```python
from build123d import *

# Parameters (mm, degrees)
BOSS_EXTRUDE1_DEPTH = 15.5
FILLET1_R           = 0.2
FILLET2_R           = 0.2
FILLET3_R           = 0.2


with BuildPart() as part:
    # Sketch1 → Boss-Extrude1 (new body)
    with BuildSketch(Plane(origin=(0, 0, 0), x_dir=(1, 0, 0), z_dir=(0, 1, 0))):
        Polygon((-0.9, 0.9), (-0.9, 2.35), (0.9, 2.35), (0.9, 0.9), (2.35, 0.9), (2.35, -0.9), (0.9, -0.9), (0.9, -2.35), (-0.9, -2.35), (-0.9, -0.9), (-2.35, -0.9), (-2.35, 0.9), align=None)
    extrude(amount=BOSS_EXTRUDE1_DEPTH)

    # Fillet1
    fillet1_edges = [part.edges().sort_by_distance(p)[0] for p in [
        (-0.9, 15.5, -1.625),
        (-1.625, 15.5, -0.9),
        (-2.35, 15.5, 0),
        (-1.625, 15.5, 0.9),
        (-0.9, 15.5, 1.625),
        (0, 15.5, 2.35),
        (0.9, 15.5, 1.625),
        (1.625, 15.5, 0.9),
        (2.35, 15.5, 0),
        (1.625, 15.5, -0.9),
        (0.9, 15.5, -1.625),
        (0, 15.5, -2.35),
    ]]
    fillet(fillet1_edges, radius=FILLET1_R)

    # Fillet2
    fillet2_edges = [part.edges().sort_by_distance(p)[0] for p in [
        (1.625, 0, -0.9),
        (2.35, 0, 0),
        (1.625, 0, 0.9),
        (0.9, 0, 1.625),
        (0, 0, 2.35),
        (-0.9, 0, 1.625),
        (-1.625, 0, 0.9),
        (-2.35, 0, 0),
        (-1.625, 0, -0.9),
        (-0.9, 0, -1.625),
        (0, 0, -2.35),
        (0.9, 0, -1.625),
    ]]
    fillet(fillet2_edges, radius=FILLET2_R)

    # Fillet3
    # the kernel refuses this fillet: 0.2 mm, written as the material it takes off along each edge
    with BuildSketch(Plane(origin=(-2.15, 15.3, 0.7), x_dir=(0, 0, 1), z_dir=(-1, 0, 0))) as fillet3_piece_1_section:
        Polygon((0, 0), (FILLET3_R, 0), (FILLET3_R, FILLET3_R), (0, FILLET3_R), align=None)
    fillet3_piece_1 = extrude(amount=FILLET3_R, mode=Mode.PRIVATE)
    fillet3_piece_1 = fillet3_piece_1 - Plane(origin=(-2.15, 15.3, 0.7), x_dir=(0, -0.7071067811865475, -0.7071067811865475), z_dir=(-1, 0, 0)) * Sphere(FILLET3_R, mode=Mode.PRIVATE)
    add(fillet3_piece_1, mode=Mode.SUBTRACT)
    with BuildSketch(Plane(origin=(-0.7, 15.3, 2.15), x_dir=(0, 0, 1), z_dir=(-1, 0, 0))) as fillet3_piece_2_section:
        Polygon((0, 0), (FILLET3_R, 0), (FILLET3_R, FILLET3_R), (0, FILLET3_R), align=None)
    fillet3_piece_2 = extrude(amount=FILLET3_R, mode=Mode.PRIVATE)
    fillet3_piece_2 = fillet3_piece_2 - Plane(origin=(-0.7, 15.3, 2.15), x_dir=(0, -0.7071067811865475, -0.7071067811865475), z_dir=(-1, 0, 0)) * Sphere(FILLET3_R, mode=Mode.PRIVATE)
    add(fillet3_piece_2, mode=Mode.SUBTRACT)
    with BuildSketch(Plane(origin=(-2.15, 15.3, -0.7), x_dir=(-1, 0, 0), z_dir=(0, 0, -1))) as fillet3_piece_3_section:
        Polygon((0, 0), (FILLET3_R, 0), (FILLET3_R, FILLET3_R), (0, FILLET3_R), align=None)
    fillet3_piece_3 = extrude(amount=FILLET3_R, mode=Mode.PRIVATE)
    fillet3_piece_3 = fillet3_piece_3 - Plane(origin=(-2.15, 15.3, -0.7), x_dir=(0.7071067811865475, -0.7071067811865475, 0), z_dir=(0, 0, -1)) * Sphere(FILLET3_R, mode=Mode.PRIVATE)
    add(fillet3_piece_3, mode=Mode.SUBTRACT)
    with BuildSketch(Plane(origin=(0.7, 15.3, 2.15), x_dir=(0, 0, 1), z_dir=(1, 0, 0))) as fillet3_piece_4_section:
        Polygon((0, 0), (FILLET3_R, 0), (FILLET3_R, -FILLET3_R), (0, -FILLET3_R), align=None)
    fillet3_piece_4 = extrude(amount=FILLET3_R, mode=Mode.PRIVATE)
    fillet3_piece_4 = fillet3_piece_4 - Plane(origin=(0.7, 15.3, 2.15), x_dir=(0, -0.7071067811865475, -0.7071067811865475), z_dir=(1, 0, 0)) * Sphere(FILLET3_R, mode=Mode.PRIVATE)
    add(fillet3_piece_4, mode=Mode.SUBTRACT)
    with BuildSketch(Plane(origin=(-0.7, 15.3, -2.15), x_dir=(0, 0, -1), z_dir=(-1, 0, 0))) as fillet3_piece_5_section:
        Polygon((0, 0), (FILLET3_R, 0), (FILLET3_R, -FILLET3_R), (0, -FILLET3_R), align=None)
    fillet3_piece_5 = extrude(amount=FILLET3_R, mode=Mode.PRIVATE)
    fillet3_piece_5 = fillet3_piece_5 - Plane(origin=(-0.7, 15.3, -2.15), x_dir=(0, -0.7071067811865475, 0.7071067811865475), z_dir=(-1, 0, 0)) * Sphere(FILLET3_R, mode=Mode.PRIVATE)
    add(fillet3_piece_5, mode=Mode.SUBTRACT)
    with BuildSketch(Plane(origin=(2.15, 15.3, 0.7), x_dir=(0, 0, 1), z_dir=(1, 0, 0))) as fillet3_piece_6_section:
        Polygon((0, 0), (FILLET3_R, 0), (FILLET3_R, -FILLET3_R), (0, -FILLET3_R), align=None)
    fillet3_piece_6 = extrude(amount=FILLET3_R, mode=Mode.PRIVATE)
    fillet3_piece_6 = fillet3_piece_6 - Plane(origin=(2.15, 15.3, 0.7), x_dir=(0, -0.7071067811865475, -0.7071067811865475), z_dir=(1, 0, 0)) * Sphere(FILLET3_R, mode=Mode.PRIVATE)
    add(fillet3_piece_6, mode=Mode.SUBTRACT)
    with BuildSketch(Plane(origin=(0.7, 15.3, -2.15), x_dir=(1, 0, 0), z_dir=(0, 0, -1))) as fillet3_piece_7_section:
        Polygon((0, 0), (FILLET3_R, 0), (FILLET3_R, -FILLET3_R), (0, -FILLET3_R), align=None)
    fillet3_piece_7 = extrude(amount=FILLET3_R, mode=Mode.PRIVATE)
    fillet3_piece_7 = fillet3_piece_7 - Plane(origin=(0.7, 15.3, -2.15), x_dir=(-0.7071067811865475, -0.7071067811865475, 0), z_dir=(0, 0, -1)) * Sphere(FILLET3_R, mode=Mode.PRIVATE)
    add(fillet3_piece_7, mode=Mode.SUBTRACT)
    with BuildSketch(Plane(origin=(2.15, 15.3, -0.7), x_dir=(1, 0, 0), z_dir=(0, 0, -1))) as fillet3_piece_8_section:
        Polygon((0, 0), (FILLET3_R, 0), (FILLET3_R, -FILLET3_R), (0, -FILLET3_R), align=None)
    fillet3_piece_8 = extrude(amount=FILLET3_R, mode=Mode.PRIVATE)
    fillet3_piece_8 = fillet3_piece_8 - Plane(origin=(2.15, 15.3, -0.7), x_dir=(-0.7071067811865475, -0.7071067811865475, 0), z_dir=(0, 0, -1)) * Sphere(FILLET3_R, mode=Mode.PRIVATE)
    add(fillet3_piece_8, mode=Mode.SUBTRACT)
    with BuildSketch(Plane(origin=(0.7, 0.2, 2.15), x_dir=(0, 0, 1), z_dir=(1, 0, 0))) as fillet3_piece_9_section:
        Polygon((0, 0), (FILLET3_R, 0), (FILLET3_R, FILLET3_R), (0, FILLET3_R), align=None)
    fillet3_piece_9 = extrude(amount=FILLET3_R, mode=Mode.PRIVATE)
    fillet3_piece_9 = fillet3_piece_9 - Plane(origin=(0.7, 0.2, 2.15), x_dir=(0, 0.7071067811865475, -0.7071067811865475), z_dir=(1, 0, 0)) * Sphere(FILLET3_R, mode=Mode.PRIVATE)
    add(fillet3_piece_9, mode=Mode.SUBTRACT)
    with BuildSketch(Plane(origin=(-0.7, 0.2, 2.15), x_dir=(0, 0, 1), z_dir=(-1, 0, 0))) as fillet3_piece_10_section:
        Polygon((0, 0), (FILLET3_R, 0), (FILLET3_R, -FILLET3_R), (0, -FILLET3_R), align=None)
    fillet3_piece_10 = extrude(amount=FILLET3_R, mode=Mode.PRIVATE)
    fillet3_piece_10 = fillet3_piece_10 - Plane(origin=(-0.7, 0.2, 2.15), x_dir=(0, 0.7071067811865475, -0.7071067811865475), z_dir=(-1, 0, 0)) * Sphere(FILLET3_R, mode=Mode.PRIVATE)
    add(fillet3_piece_10, mode=Mode.SUBTRACT)
    with BuildSketch(Plane(origin=(2.15, 0.2, 0.7), x_dir=(0, 0, 1), z_dir=(1, 0, 0))) as fillet3_piece_11_section:
        Polygon((0, 0), (FILLET3_R, 0), (FILLET3_R, FILLET3_R), (0, FILLET3_R), align=None)
    fillet3_piece_11 = extrude(amount=FILLET3_R, mode=Mode.PRIVATE)
    fillet3_piece_11 = fillet3_piece_11 - Plane(origin=(2.15, 0.2, 0.7), x_dir=(0, 0.7071067811865475, -0.7071067811865475), z_dir=(1, 0, 0)) * Sphere(FILLET3_R, mode=Mode.PRIVATE)
    add(fillet3_piece_11, mode=Mode.SUBTRACT)
    with BuildSketch(Plane(origin=(-2.15, 0.2, 0.7), x_dir=(0, 0, 1), z_dir=(-1, 0, 0))) as fillet3_piece_12_section:
        Polygon((0, 0), (FILLET3_R, 0), (FILLET3_R, -FILLET3_R), (0, -FILLET3_R), align=None)
    fillet3_piece_12 = extrude(amount=FILLET3_R, mode=Mode.PRIVATE)
    fillet3_piece_12 = fillet3_piece_12 - Plane(origin=(-2.15, 0.2, 0.7), x_dir=(0, 0.7071067811865475, -0.7071067811865475), z_dir=(-1, 0, 0)) * Sphere(FILLET3_R, mode=Mode.PRIVATE)
    add(fillet3_piece_12, mode=Mode.SUBTRACT)
    with BuildSketch(Plane(origin=(2.15, 0.2, -0.7), x_dir=(1, 0, 0), z_dir=(0, 0, -1))) as fillet3_piece_13_section:
        Polygon((0, 0), (FILLET3_R, 0), (FILLET3_R, FILLET3_R), (0, FILLET3_R), align=None)
    fillet3_piece_13 = extrude(amount=FILLET3_R, mode=Mode.PRIVATE)
    fillet3_piece_13 = fillet3_piece_13 - Plane(origin=(2.15, 0.2, -0.7), x_dir=(-0.7071067811865475, 0.7071067811865475, 0), z_dir=(0, 0, -1)) * Sphere(FILLET3_R, mode=Mode.PRIVATE)
    add(fillet3_piece_13, mode=Mode.SUBTRACT)
    with BuildSketch(Plane(origin=(-2.15, 0.2, -0.7), x_dir=(-1, 0, 0), z_dir=(0, 0, -1))) as fillet3_piece_14_section:
        Polygon((0, 0), (FILLET3_R, 0), (FILLET3_R, -FILLET3_R), (0, -FILLET3_R), align=None)
    fillet3_piece_14 = extrude(amount=FILLET3_R, mode=Mode.PRIVATE)
    fillet3_piece_14 = fillet3_piece_14 - Plane(origin=(-2.15, 0.2, -0.7), x_dir=(0.7071067811865475, 0.7071067811865475, 0), z_dir=(0, 0, -1)) * Sphere(FILLET3_R, mode=Mode.PRIVATE)
    add(fillet3_piece_14, mode=Mode.SUBTRACT)
    with BuildSketch(Plane(origin=(0.7, 0.2, -2.15), x_dir=(1, 0, 0), z_dir=(0, 0, -1))) as fillet3_piece_15_section:
        Polygon((0, 0), (FILLET3_R, 0), (FILLET3_R, FILLET3_R), (0, FILLET3_R), align=None)
    fillet3_piece_15 = extrude(amount=FILLET3_R, mode=Mode.PRIVATE)
    fillet3_piece_15 = fillet3_piece_15 - Plane(origin=(0.7, 0.2, -2.15), x_dir=(-0.7071067811865475, 0.7071067811865475, 0), z_dir=(0, 0, -1)) * Sphere(FILLET3_R, mode=Mode.PRIVATE)
    add(fillet3_piece_15, mode=Mode.SUBTRACT)
    with BuildSketch(Plane(origin=(-0.7, 0.2, -2.15), x_dir=(0, 0, -1), z_dir=(-1, 0, 0))) as fillet3_piece_16_section:
        Polygon((0, 0), (FILLET3_R, 0), (FILLET3_R, FILLET3_R), (0, FILLET3_R), align=None)
    fillet3_piece_16 = extrude(amount=FILLET3_R, mode=Mode.PRIVATE)
    fillet3_piece_16 = fillet3_piece_16 - Plane(origin=(-0.7, 0.2, -2.15), x_dir=(0, 0.7071067811865475, 0.7071067811865475), z_dir=(-1, 0, 0)) * Sphere(FILLET3_R, mode=Mode.PRIVATE)
    add(fillet3_piece_16, mode=Mode.SUBTRACT)
    with BuildSketch(Plane(origin=(2.35, 0.2, -0.9), x_dir=(-1, 0, 0), z_dir=(0, 1, 0)), Plane(origin=(2.35, 0.2, 0.9), x_dir=(0, 0, -1), z_dir=(0, 1, 0)), Plane(origin=(0.9, 0.2, 2.35), x_dir=(0, 0, -1), z_dir=(0, 1, 0)), Plane(origin=(-0.9, 0.2, -2.35), x_dir=(0, 0, 1), z_dir=(0, 1, 0)), Plane(origin=(0.9, 0.2, -2.35), x_dir=(-1, 0, 0), z_dir=(0, 1, 0))) as fillet3_piece_17:
        with BuildLine():
            CenterArc((FILLET3_R, FILLET3_R), FILLET3_R, 180, 90)
            Line((0, FILLET3_R), (0, 0))
            Line((0, 0), (FILLET3_R, 0))
        make_face()
    extrude(amount=15.1, mode=Mode.SUBTRACT)
    with BuildSketch(Plane(origin=(-0.9, 0.2, 2.35), x_dir=(0, 0, -1), z_dir=(0, 1, 0)), Plane(origin=(-2.35, 0.2, 0.9), x_dir=(0, 0, -1), z_dir=(0, 1, 0)), Plane(origin=(-2.35, 0.2, -0.9), x_dir=(1, 0, 0), z_dir=(0, 1, 0))) as fillet3_piece_18:
        with BuildLine():
            CenterArc((FILLET3_R, -FILLET3_R), FILLET3_R, 90, 90)
            Line((0, -FILLET3_R), (0, 0))
            Line((0, 0), (FILLET3_R, 0))
        make_face()
    extrude(amount=15.1, mode=Mode.SUBTRACT)


solid = part.part
```
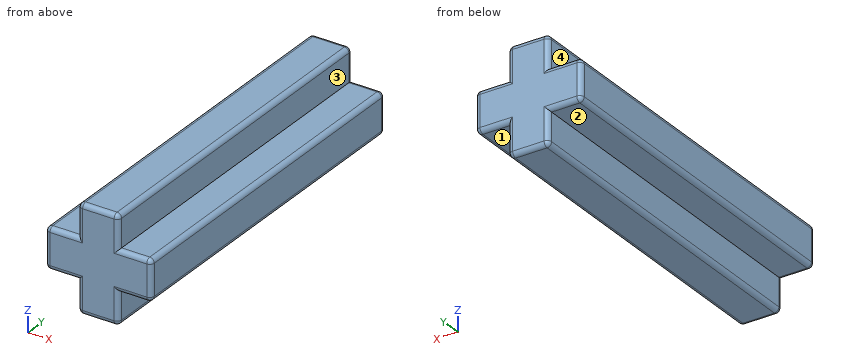
Geometry check sheet. Reference: the model listing, model coordinates, mm. Face numbers are marked on the shaded views. A direction names the side the tool comes from. Round coordinates to 2 decimals unless told otherwise and drop trailing zeros. Loops run counter-clockwise (first coordinate to the right, second up) from the corner with the lowest first, then second, coordinate; pieces in that order, holes last. Notation, with made-up numbers: (19, 31) - (56, 31) arc R36 ccw to (56, 67) - close; hole circle Ø11 at (27, 29). An arc over 180 degrees is marked (long way). Use a Markdown table: item, result.
Q1. Material ranges on line 1 (X direction, y = 5.5, z = 1.6); line 2 (Z direction, x = 0.85, y = 9.5), recorded low to high.
Solutions:
| item | result |
|---|---|
| line 1 | x = -0.9 to 0.9 |
| line 2 | z = -2.28 to 2.28 |
Q2. Cross-section at B-B on z = -1.55. Record the cut outline in (x, y), plus the area to 3 significant figures.
Solutions:
| item | result |
|---|---|
| outline | (-0.9, 0.2) arc R0.2 ccw to (-0.7, 0) - (0.7, 0) arc R0.2 ccw to (0.9, 0.2) - (0.9, 15.3) arc R0.2 ccw to (0.7, 15.5) - (-0.7, 15.5) arc R0.2 ccw to (-0.9, 15.3) - close |
| area | 27.9 mm2 |
Q3. Cross-section at A-A on x = 1.25. Record the cut outline in (y, z), plus the area to 3 significant figures.
Solutions:
| item | result |
|---|---|
| outline | (0, -0.7) arc R0.2 ccw to (0.2, -0.9) - (15.3, -0.9) arc R0.2 ccw to (15.5, -0.7) - (15.5, 0.7) arc R0.2 ccw to (15.3, 0.9) - (0.2, 0.9) arc R0.2 ccw to (0, 0.7) - close |
| area | 27.9 mm2 |
Q4. Access from +Z, -Z, +X, -X, +Y, -Y to the whole of each face (thin tool, end or side, straight path). Record for the marked faces 1, 2, 3 and 4.
Solutions:
| item | result |
|---|---|
| face 1 | -Z, +X, +Y, -Y |
| face 2 | -Z, -X, +Y, -Y |
| face 3 | +Z, +X, +Y, -Y |
| face 4 | +Z, -X, +Y, -Y |
Q5. Cross-section at C-C on y = 9.5. Record the cut outline in (x, z).
Solutions:
| item | result |
|---|---|
| outline | (-2.35, -0.7) arc R0.2 ccw to (-2.15, -0.9) - (-0.9, -0.9) - (-0.9, -2.15) arc R0.2 ccw to (-0.7, -2.35) - (0.7, -2.35) arc R0.2 ccw to (0.9, -2.15) - (0.9, -0.9) - (2.15, -0.9) arc R0.2 ccw to (2.35, -0.7) - (2.35, 0.7) arc R0.2 ccw to (2.15, 0.9) - (0.9, 0.9) - (0.9, 2.15) arc R0.2 ccw to (0.7, 2.35) - (-0.7, 2.35) arc R0.2 ccw to (-0.9, 2.15) - (-0.9, 0.9) - (-2.15, 0.9) arc R0.2 ccw to (-2.35, 0.7) - close |
Q6. Go/stop test with flat-tipped pins: P1, Ø1.5, axis at x = -1, z = 1, coming from the +Y side; P2, Ø1, axis at y = 7.5, z = 1.5, coming from the +X side; P3, Ø0.6, axis at y = 9, z = -1.5, coming from the -X side; P4, Ø1, axis at x = -1.5, y = 5.5, coming from the -Z side. Record where each tip stops, or that it passes through.
Solutions:
| item | result |
|---|---|
| P1 | stops at y = 15.5 |
| P2 | stops at x = 0.9 |
| P3 | stops at x = -0.9 |
| P4 | stops at z = -0.9 |
